from build123d import *

# Parameters (mm, degrees)
F0_W     = 100
F0_H     = 80
F0_W_2   = 20
F0_H_2   = 30
F0_H_3   = 50
F0_H_4   = 5
F1_DEPTH = 2.5
F2_SIZE2 = 3.570407
F2_SIZE  = 4.99999


# Not quite as in the source:
# - a fillet or chamfer is up to 0.001 mm smaller than in the source, because OpenCascade refuses the exact size


with BuildPart() as f1:
    # F0 (on Right) → F1 (new body, symmetric)
    with BuildSketch(Plane.YZ):
        with Locations((-50, 40)):
            Rectangle(F0_W, F0_H)
        with Locations((-70, 40)):
            Rectangle(F0_W_2, F0_H_2, mode=Mode.SUBTRACT)
        with Locations((-50, 105)):
            Rectangle(F0_W, F0_H_3)
        with Locations((-50, -2.5)):
            Rectangle(F0_W, F0_H_4)
    extrude(amount=F1_DEPTH, both=True)

    # F2 (size 5 and 3.5704168108 in the source; OpenCascade refuses exactly that, so slightly less here)
    f2_edges = [f1.edges().sort_by_distance(p)[0] for p in [
        (2.5, -50, 130),
    ]]
    f2_side = f1.faces().sort_by_distance((0, -50, 130))[0]
    chamfer(f2_edges, length=F2_SIZE, length2=F2_SIZE2, reference=f2_side)


solid = f1.part
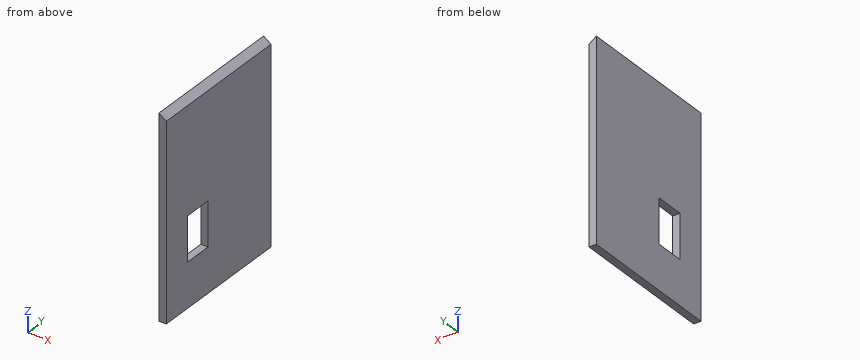
Geometry check sheet. Reference: the model listing, model coordinates, mm. Give positions to 0.01 mm unless a question says otherwise; leave off trailing zeros. Write each loop counter-clockwise with the first axis right and the second up, starting at its lowest first coordinate (ties: lowest second). Pieces come first, ordered by that corner, then holes. Notation, with made-up numbers: M 89.5,78.25 L 113.5,78.25 A22 ccw 113.5,107.25 Z; hole C 14.25,-1 d3. An arc over 180 degrees is marked long. One line per question, with ' | ' between items.
1. Cross-section at B-B (x = -0.45). Enter the section's corners in (y, z), plus the area to 3 significant figures.
Ans:
outline: M -100,-5 L 0,-5 L 0,128.54 L -100,128.54 Z; hole M -80,25 L -60,25 L -60,55 L -80,55 Z | area: 12,800 mm2
2. Gauge pin test, flat ends, axial feed: pin 1 (1.5 mm diameter, centred on x = 1, z = 33.5, fed in from +Y); pin 2 (1.5 mm diameter, centred on x = 0.5, y = -74.5, fed in from +Z). Record the tip position at first contact, or that the pin passes through.
Ans:
pin 1: y = 0 | pin 2: z = 128.39
3. Scan lines: line 1 along Y through (x, z) = (-0.8, 44); line 2 along Z through (x, y) = (-0.2, -64.5); line 3 along Z through (x, y) = (-1, -4). Record each from-to range of solid material in increasing order. Write a range as from..to.
Ans:
line 1: -100..-80, -60..0 | line 2: -5..25, 55..128.36 | line 3: -5..128.93
4. Cross-section at A-A (z = 31). Enter the section's corners in (x, y).
Ans:
outline: M -2.5,-100 L 2.5,-100 L 2.5,-80 L -2.5,-80 Z; M -2.5,-60 L 2.5,-60 L 2.5,0 L -2.5,0 Z
